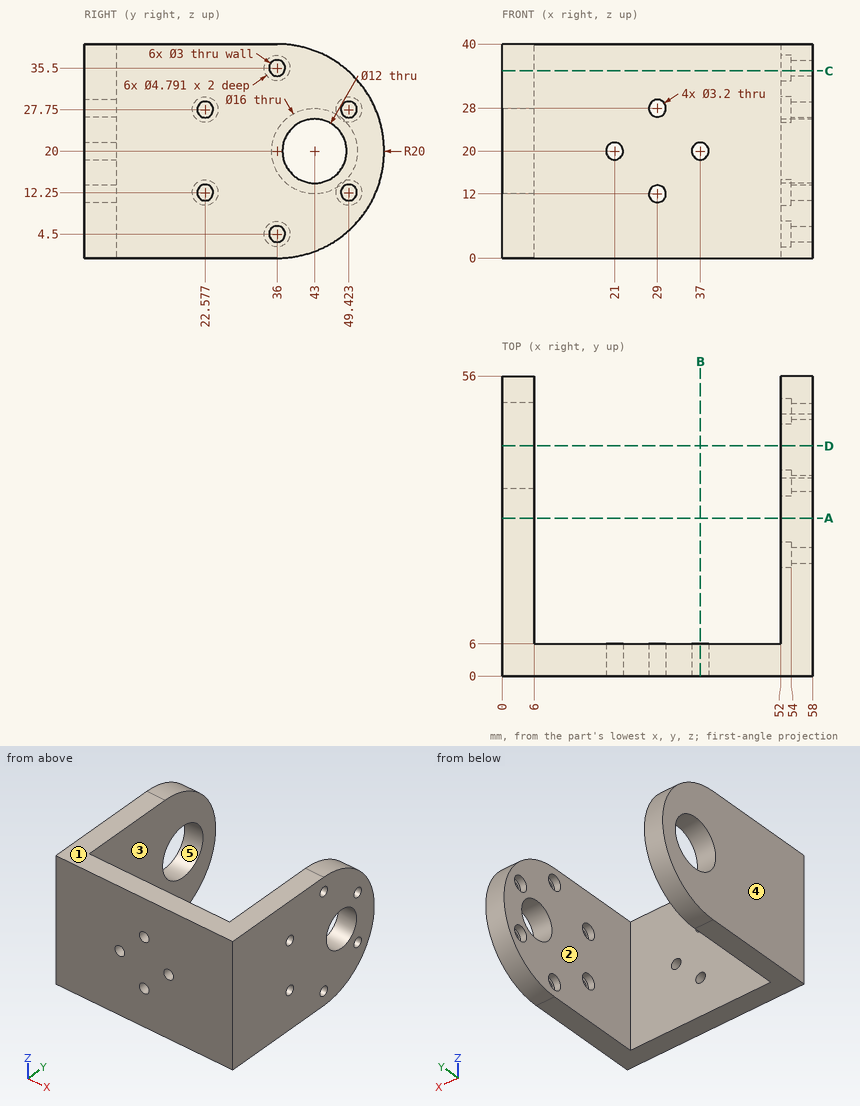
Job drawing, mm, ordinate dimensions from the low corner. One solid piece. A direction names the side the tool comes from. Round coordinates to 2 decimals unless told otherwise and drop trailing zeros. Loops run counter-clockwise (first coordinate to the right, second up) from the corner with the lowest first, then second, coordinate; pieces in that order, holes last. Notation, with made-up numbers: (-16, 16) -> (28, 16) arc R27 cw to (28, 41) -> close; hole circle Ø1 at (-10.5, -35). An arc over 180 degrees is marked (long way). One line per item, written item: value. Start each with the question number.
Q1. Drop flat-ended pins along their axis: pin 1 Ø10 at (x, y) = (14, 46.5) entering from +Z; pin 2 Ø4 at (x, z) = (33, 19) entering from +Y. Give the stop position or say it passes through.
Q2. Probe line 1 along X through (y, z) = (35, 19); line 2 along Y through (x, z) = (53.3, 12.25); line 3 along X through (y, z) = (50, 14.5). List the from-to ranges inside material, lowest first.
Q3. 3-axis set-ups, long thin cutter, end or side, ignore diameter. For the marked faces 1 and 2: which of +Z, -Z, +X, -X, +Y, -Y reach the whole face in a straight line?
Q4. Cut at C-C on z = 35. List the corners of the cut face in (x, y) (1 decimal), plus the area to 3 significant figures.
Q5. Cut at A-A on y = 29.5. List the corners of the cut face in (x, z), plus the area to 3 significant figures.
Q6. Cut at B-B on x = 37. List the corners of the cut face in (y, z).
Q7. Two-plate mould, pull along X, no slides. Class the marked faces 3, 4 and 5: released by +X, released by -X, zero draft, split by the parting line, or undercut.
Q8. Cut at D-D on y = 43. List the corners of the cut face in (x, z) (1 decimal).
Computed:
1. pin 1: through
1. pin 2: y = 6
2. line 1: 0 to 6, 52 to 58
2. line 2: 0 to 20.18, 24.97 to 47.03, 51.82 to 54.44
2. line 3: 0 to 6, 54 to 58
3. face 1: +Z, +X, -X, +Y, -Y
3. face 2: +Z, -Z, +Y
4. outline: (0, 0) -> (58, 0) -> (58, 34.6) -> (54, 34.6) -> (54, 33.7) -> (52, 33.7) -> (52, 6) -> (6, 6) -> (6, 49.2) -> (0, 49.2) -> close; (52, 38.3) -> (54, 38.3) -> (54, 37.4) -> (58, 37.4) -> (58, 49.2) -> (52, 49.2) -> close
4. area: 846 mm²
5. outline: (0, 0) -> (6, 0) -> (6, 40) -> (0, 40) -> close; (52, 0) -> (58, 0) -> (58, 40) -> (52, 40) -> close
5. area: 480 mm²
6. outline: (0, 0) -> (6, 0) -> (6, 18.4) -> (0, 18.4) -> close; (0, 21.6) -> (6, 21.6) -> (6, 40) -> (0, 40) -> close
7. face 3: undercut
7. face 4: released by -X
7. face 5: zero draft
8. outline: (0, 1.3) -> (6, 1.3) -> (6, 12) -> (0, 12) -> close; (0, 28) -> (6, 28) -> (6, 38.7) -> (0, 38.7) -> close; (52, 1.3) -> (58, 1.3) -> (58, 14) -> (52, 14) -> close; (52, 26) -> (58, 26) -> (58, 38.7) -> (52, 38.7) -> close
